Geometry: final body of the model. Coordinates: model frame, mm. A direction names the side the tool comes from. Round coordinates to 2 decimals unless told otherwise and drop trailing zeros. Loops run counter-clockwise (first coordinate to the right, second up) from the corner with the lowest first, then second, coordinate; pieces in that order, holes last. Notation, with made-up numbers: (58.5, -31.75) - (74.5, -31.75) arc R25 ccw to (74.5, 7.25) - close; hole circle Ø9 at (25, -26). An arc over 180 degrees is marked (long way). Write item = value, one per line. Start each with the question number.
Item 1: Section D-D (z = 5.5). Return loops of the section in (x, y) (3 decimals).
Item 2: Section B-B (x = 0). Return loops of the section in (y, z) (1 decimal), plus the area to 3 significant figures.
Item 3: Line query: line 1 (X direction, y = 36, z = 24); line 2 (Z direction, x = -6.5, y = -12); line 3 (Y direction, x = 0, z = 13.5) (3 decimals). Output: solid intervals per line, ascending. Write a range as from..to.
Item 4: Section C-C (z = 31.5). Return loops of the section in (x, y).
Item 5: First-contact query: pin 1 (8.5 mm diameter, centred on y = -32.5, z = 29, fed in from -X); pin 2 (3 mm diameter, centred on x = -4.5, y = 31, fed in from -Z); pin 3 (8.5 mm diameter, centred on y = -23, z = 27.5, fed in from +X). Flat tips, straight axial feed; report the tip coordinate or a pass-through.
Item 6: Access query for faces 1 (the cylindrical face through (0.05, -37.58, 42.69)), 2 (the flat face through (-0.049, 19.756, 28.873)). Directions: +Z, -Z, +X, -X, +Y, -Y. A direction counts if a zero-diameter tool reaches every point of the face in a straight line with its end or side. Return the directions, or none.
Item 7: Draft query along X for faces 3 (the cylindrical face through (-8.57, -1.13, 10.64)), 4 (the flat face through (-10.2, -0.2, 21)), 5 (the conical face through (-15.5, 0.3, 10.4)). Return one class per face: pulls with the +X half, pulls with the -X half, needs draft (parallel to the pull), parting line crosses it, or undercut.
Item 8: Section A-A (y = 0). Return loops of the section in (x, z) (3 decimals).
from build123d import *

# Parameters (mm, degrees)
PAD_DEPTH = 3.5


with BuildPart() as pad:
    # Sketch001 → Pad (new body, symmetric)
    with BuildSketch(Plane.YZ):
        with BuildLine():
            Line((11, 0), (11, 21))
            Line((11, 21), (17, 21))
            Line((17, 21), (22.589568, 36.968909))
            ThreePointArc((40.381508, 26.562289), (37.80128, 42.563467), (22.589568, 36.968909))
            Line((17, 0), (40.381508, 26.562289))
            Line((11, 0), (17, 0))
        make_face()
        with BuildLine():
            Line((-40.381517, 26.562321), (-17.000046, 0))
            Line((-17.000046, 0), (-11.000046, 0))
            Line((-11.000046, 0), (-11.000046, 21))
            Line((-11.000046, 21), (-17.000046, 21))
            Line((-17.000046, 21), (-22.589566, 36.968926))
            ThreePointArc((-22.589566, 36.968926), (-37.801272, 42.563494), (-40.381517, 26.562321))
        make_face()
    extrude(amount=PAD_DEPTH, both=True)


with BuildPart() as obj1:
    # Sketch → Revolution (revolve)
    with BuildSketch(Plane.YZ):
        Polygon((10, 0), (8.645, 0.78231), (8.645, 20.21769), (10, 21), (15, 21), (16, 0), align=None)
    revolve(axis=Axis((0, 0, 0), (0, 0, 1)))

    # Fusion: union Pad
    add(pad.part)


solid = obj1.part
Taken from the geometry:
q1.outline = (-3.5, -21.841) - (3.5, -21.841) - (3.5, -15.344) arc R15.738 ccw to (3.5, 15.344) - (3.5, 21.841) - (-3.5, 21.841) - (-3.5, 15.344) arc R15.738 ccw to (-3.5, -15.344) - close; hole circle Ø17.29 at (0, 0)
q2.outline = (-40.4, 26.6) - (-17, 0) - (-10, 0) - (-8.6, 0.8) - (-8.6, 20.2) - (-10, 21) - (-17, 21) - (-22.6, 37) arc R10.5 ccw (long way) to start; (8.6, 0.8) - (10, 0) - (17, 0) - (40.4, 26.6) arc R10.5 ccw (long way) to (22.6, 37) - (17, 21) - (10, 21) - (8.6, 20.2) - close
q2.area = 1,610 mm^2
q3.line_1 = -3.5..3.5
q3.line_2 = 0..21
q3.line_3 = -28.883..-8.645, 8.645..28.883
q4.outline = (-3.5, -42.81) - (3.5, -42.81) - (3.5, -20.68) - (-3.5, -20.68) - close; (-3.5, 20.68) - (3.5, 20.68) - (3.5, 42.81) - (-3.5, 42.81) - close
q5.pin_1 = -3.5
q5.pin_2 = 14.63
q5.pin_3 = 3.5
q6.face_1 = +X, -X
q6.face_2 = +Z, +X, -X
q7.face_3 = undercut
q7.face_4 = needs draft
q7.face_5 = pulls with the -X half
q8.outline = (-16, 0) - (-10, 0) - (-8.645, 0.782) - (-8.645, 20.218) - (-10, 21) - (-15, 21) - close; (8.645, 0.782) - (10, 0) - (16, 0) - (15, 21) - (10, 21) - (8.645, 20.218) - close
